Check sheet for the modelled part. Datum: model origin and axes. Units: mm. Give positions to 0.01 mm unless a question says otherwise; leave off trailing zeros. Write each loop counter-clockwise with the first axis right and the second up, starting at its lowest first coordinate (ties: lowest second). Pieces come first, ordered by that corner, then holes. Notation, with made-up numbers: (-19, 88) - (34, 88) arc R27 ccw to (34, 126) - close; hole circle Ø5 at (-4.75, -7). An arc over 180 degrees is marked (long way). Return JSON: item names as keys, results as strings. Group by question number.
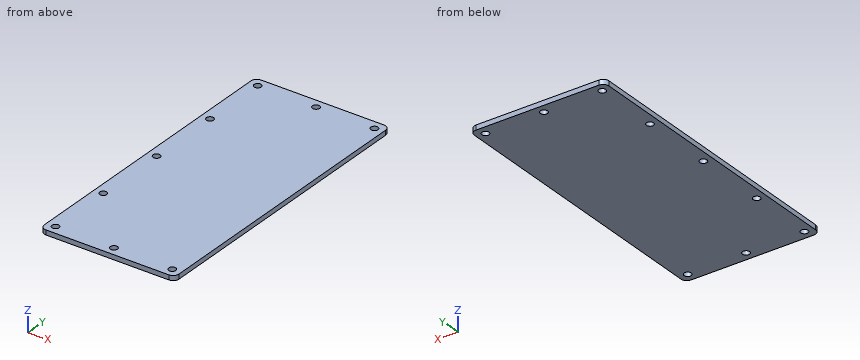
```python
from build123d import *

# Parameters (mm, degrees)
EXTRUDE_1_DEPTH     = 8
SKETCH_2_R          = 6
CUT_EXTRUDE_1_DEPTH = 10


with BuildPart() as part:
    # 草图1 → 凸台-拉伸1 (new body)
    with BuildSketch(Plane.XY):
        with BuildLine():
            Line((10, 0), (215, 0))
            ThreePointArc((215, 0), (222.071067812, 2.928932188), (225, 10))
            Line((225, 10), (225, 486))
            ThreePointArc((225, 486), (222.071067812, 493.071067812), (215, 496))
            Line((215, 496), (10, 496))
            ThreePointArc((10, 496), (2.928932188, 493.071067812), (0, 486))
            Line((0, 486), (0, 10))
            ThreePointArc((0, 10), (2.928932188, 2.928932188), (10, 0))
        make_face()
    extrude(amount=EXTRUDE_1_DEPTH)

    # 草图2 → 切除-拉伸1 (cut)
    with BuildSketch(Plane.XY.offset(8)):
        with Locations((112.5, 481)):
            Circle(SKETCH_2_R)
        with Locations((210, 481)):
            Circle(SKETCH_2_R)
        with Locations((15, 481)):
            Circle(SKETCH_2_R)
        with Locations((15, 15)):
            Circle(SKETCH_2_R)
        with Locations((210, 15)):
            Circle(SKETCH_2_R)
        with Locations((112.5, 15)):
            Circle(SKETCH_2_R)
        with Locations((15, 248)):
            Circle(SKETCH_2_R)
        with Locations((15, 371)):
            Circle(SKETCH_2_R)
        with Locations((15, 125)):
            Circle(SKETCH_2_R)
    extrude(amount=-CUT_EXTRUDE_1_DEPTH, mode=Mode.SUBTRACT)


solid = part.part
```
Item 1: Section check A-A on y = 371. Record the cut outline in (x, z).
Item 2: Section check B-B on y = 481. Record the cut outline in (x, z).
Item 3: Depth check by flat-ended pin: pin 1 (14 mm diameter, centred on x = 210, y = 481, fed in from +Z). Enter the tip coordinate at first touch or a pass-through.
Item 4: Material ranges on line 1 along Y through (x, z) = (210, 3.75); line 2 along Y through (x, z) = (15, 5.5); line 3 along X through (y, z) = (481, 3.25), recorded low to high. Write a range as from..to.
Reply:
{
 "1": {"outline": "(0, 0) - (9, 0) - (9, 8) - (0, 8) - close; (21, 0) - (225, 0) - (225, 8) - (21, 8) - close"},
 "2": {"outline": "(0, 0) - (9, 0) - (9, 8) - (0, 8) - close; (21, 0) - (106.5, 0) - (106.5, 8) - (21, 8) - close; (118.5, 0) - (204, 0) - (204, 8) - (118.5, 8) - close; (216, 0) - (225, 0) - (225, 8) - (216, 8) - close"},
 "3": {"pin 1": "z = 8"},
 "4": {"line 1": "0..9, 21..475, 487..496", "line 2": "0..9, 21..119, 131..242, 254..365, 377..475, 487..496", "line 3": "0..9, 21..106.5, 118.5..204, 216..225"}
}
